Geometry: final body of the model. Coordinates: model frame, mm. A direction names the side the tool comes from. Round coordinates to 2 decimals unless told otherwise and drop trailing zeros. Loops run counter-clockwise (first coordinate to the right, second up) from the corner with the lowest first, then second, coordinate; pieces in that order, holes last. Notation, with made-up numbers: M 38,-26.75 L 64,-26.75 A31 ccw 64,-0.75 Z; hole C 34.25,-17 d1. An arc over 180 degrees is marked long. Write each question's results on one line, items separated by ' | '.
```python
from build123d import *

# Parameters (mm, degrees)
SZKIC1_W                         = 25.6
SZKIC1_H                         = 10
DODANIE_WYCI_GNI_CIE1_DEPTH      = 5
SZKIC2_R                         = 1.75
WYTNIJ_WYCI_GNI_CIE1_DEPTH       = 5
SZKIC3_W                         = 25.6
SZKIC3_H                         = 5
DODANIE_WYCI_GNI_CIE2_DEPTH      = 5
SZKIC4_W                         = 25.6
SZKIC4_H                         = 5
DODANIE_WYCI_GNI_CIE3_DEPTH      = 17
SZKIC5_R                         = 1.75
WYTNIJ_WYCI_GNI_CIE2_DEPTH       = 20
SZKIC6_W                         = 2
SZKIC6_H                         = 15
WYTNIJ_WYCI_GNI_CIE3_DEPTH       = 28.346663416
DODANIE_WYCI_GNI_CIE4_DEPTH      = 0.5
DODANIE_WYCI_GNI_CIE4_DEPTH_BACK = 7.5
SZKIC8_R                         = 1.75
WYTNIJ_WYCI_GNI_CIE4_DEPTH       = 48.531147682
SZKIC9_W                         = 37
SZKIC9_H                         = 6
DODANIE_WYCI_GNI_CIE5_DEPTH      = 20.5
SZKIC10_W                        = 37
SZKIC10_H                        = 6
SZKIC10_R                        = 1.75
DODANIE_WYCI_GNI_CIE6_DEPTH      = 5
SZKIC11_W                        = 16.1
SZKIC11_H                        = 5
DODANIE_WYCI_GNI_CIE7_DEPTH      = 15
SFAZOWANIE2_SIZE                 = 7.5
SFAZOWANIE2_SIZE2                = 2.009618943


with BuildPart() as part:
    # Szkic1 → Dodanie-wyciągnięcie1 (new body)
    with BuildSketch(Plane.XY):
        Rectangle(SZKIC1_W, SZKIC1_H)
    extrude(amount=DODANIE_WYCI_GNI_CIE1_DEPTH)

    # Szkic2 → Wytnij-wyciągnięcie1 (cut)
    with BuildSketch(Plane.XY.offset(5)):
        with Locations((-6, 0)):
            Circle(SZKIC2_R)
        with Locations((6, 0)):
            Circle(SZKIC2_R)
    extrude(amount=-WYTNIJ_WYCI_GNI_CIE1_DEPTH, mode=Mode.SUBTRACT)

    # Szkic3 → Dodanie-wyciągnięcie2 (add)
    with BuildSketch(Plane(origin=(0, 5, 0), x_dir=(1, 0, 0), z_dir=(0, 1, 0))):
        with Locations((0, -2.5)):
            Rectangle(SZKIC3_W, SZKIC3_H)
    extrude(amount=DODANIE_WYCI_GNI_CIE2_DEPTH)

    # Szkic4 → Dodanie-wyciągnięcie3 (add)
    with BuildSketch(Plane(origin=(0, 0, 0), x_dir=(-1, 0, 0), z_dir=(0, 0, -1))):
        with Locations((0, 7.5)):
            Rectangle(SZKIC4_W, SZKIC4_H)
    extrude(amount=DODANIE_WYCI_GNI_CIE3_DEPTH)

    # Szkic5 → Wytnij-wyciągnięcie2 (cut)
    with BuildSketch(Plane(origin=(0, 10, 0), x_dir=(1, 0, 0), z_dir=(0, 1, 0))):
        with Locations(Location((-0.8, 12, 0), (0, 0, 180))):
            Circle(SZKIC5_R)
    extrude(amount=-WYTNIJ_WYCI_GNI_CIE2_DEPTH, mode=Mode.SUBTRACT)

    # Szkic6 → Wytnij-wyciągnięcie3 (cut, through all)
    with BuildSketch(Plane.XY.offset(5)):
        with Locations((11.8, 2.5)):
            Rectangle(SZKIC6_W, SZKIC6_H)
    extrude(amount=-WYTNIJ_WYCI_GNI_CIE3_DEPTH, mode=Mode.SUBTRACT)

    # Szkic7 → Dodanie-wyciągnięcie4 (add, two sides: drawn at the far end of the back side and taken through both)
    with BuildSketch(Plane(origin=(10.8, 0, 0), x_dir=(0, 0, -1), z_dir=(1, 0, 0)).offset(-DODANIE_WYCI_GNI_CIE4_DEPTH_BACK)):
        Polygon((-5, 10), (17, 10), (17, 20), (-8, 40), (-16, 40), (-20, 25), (-20, 5), (-5, 5), align=None)
    extrude(amount=DODANIE_WYCI_GNI_CIE4_DEPTH + DODANIE_WYCI_GNI_CIE4_DEPTH_BACK)

    # Szkic8 → Wytnij-wyciągnięcie4 (cut, through all)
    with BuildSketch(Plane.ZY.offset(-3.3)):
        with Locations((12.5, 15)):
            Circle(SZKIC8_R)
        with Locations((12.5, 36.7)):
            Circle(SZKIC8_R)
        with Locations((-11.5, 15)):
            Circle(SZKIC8_R)
    extrude(amount=-WYTNIJ_WYCI_GNI_CIE4_DEPTH, mode=Mode.SUBTRACT)

    # Szkic9 → Dodanie-wyciągnięcie5 (add)
    with BuildSketch(Plane(origin=(10.8, 0, 0), x_dir=(0, 0, -1), z_dir=(1, 0, 0))):
        with Locations((-1.5, 8)):
            Rectangle(SZKIC9_W, SZKIC9_H)
    extrude(amount=DODANIE_WYCI_GNI_CIE5_DEPTH)

    # Szkic10 → Dodanie-wyciągnięcie6 (add)
    # profile 1 of 2: a face of its own
    with BuildSketch(Plane(origin=(31.3, 0, 0), x_dir=(0, 0, -1), z_dir=(1, 0, 0))):
        with Locations((-1.5, 8)):
            Rectangle(SZKIC10_W, SZKIC10_H)
    # profile 2 of 2: a face of its own
    with BuildSketch(Plane(origin=(31.3, 0, 0), x_dir=(0, 0, -1), z_dir=(1, 0, 0))):
        Polygon((-8, 40), (-16, 40), (-20, 25), (-20, 11), (17, 11), (17, 20), align=None)
        with Locations(Location((-12.5, 15, 0), (0, 0, 180))):
            Circle(SZKIC10_R, mode=Mode.SUBTRACT)
        with Locations(Location((-12.5, 36.7, 0), (0, 0, 180))):
            Circle(SZKIC10_R, mode=Mode.SUBTRACT)
        with Locations(Location((11.5, 15, 0), (0, 0, 180))):
            Circle(SZKIC10_R, mode=Mode.SUBTRACT)
    extrude(amount=DODANIE_WYCI_GNI_CIE6_DEPTH)

    # Szkic11 → Dodanie-wyciągnięcie7 (add)
    with BuildSketch(Plane.XY.offset(5)):
        with Locations((-4.75, 7.5)):
            Rectangle(SZKIC11_W, SZKIC11_H)
    extrude(amount=DODANIE_WYCI_GNI_CIE7_DEPTH)

    # Sfazowanie2
    sfazowanie2_edges = [part.edges().sort_by_distance(p)[0] for p in [
        (36.3, 5, 1.5),
    ]]
    sfazowanie2_side = [part.faces().sort_by_distance(p)[0] for p in [
        (12.712207968, 5, 1.507036511),
    ]]
    chamfer(sfazowanie2_edges, length=SFAZOWANIE2_SIZE, length2=SFAZOWANIE2_SIZE2, reference=sfazowanie2_side[0])


solid = part.part
```
1. Pin query (flat end, axial travel): P1, Ø8, axis at y = 29, z = 3, coming from the -X side; P2, Ø4, axis at x = -0.5, y = 18, coming from the +Z side; P3, Ø6, axis at x = -5, z = 7, coming from the +Y side; P4, Ø8, axis at x = 29, z = -11, coming from the -Y side. Return the tip coordinate at first contact, or that it passes through.
Answer key:
P1: stops at x = 3.3 | P2: passes through | P3: stops at y = 10 | P4: stops at y = 5
2. Access query for faces 1 (the face through (11.3, 22, 6)), 2 (the face through (36.3, 20, 6)). Directions: +Z, -Z, +X, -X, +Y, -Y. A direction counts if a zero-diameter tool reaches every point of the face in a straight line with its end or side. Return the directions, or none.
Answer key:
face 1: +Z, -Z, +Y | face 2: +Z, -Z, +X, +Y, -Y
3. Section A-A (x = 6). Output: boundary loops of the cut face in (y, z).
Answer key:
outline: M -5,0 L -1.75,0 L -1.75,5 L -5,5 Z; M 1.75,0 L 5,0 L 5,-17 L 20,-17 L 40,8 L 40,16 L 25,20 L 5,20 L 5,5 L 1.75,5 Z; hole C 15,-11.5 d3.5; hole C 15,12.5 d3.5; hole C 36.7,12.5 d3.5
4. Section C-C (z = -12). Output: boundary loops of the cut face in (x, y).
Answer key:
outline: M -12.8,5 L -2.55,5 L -2.55,10 L -12.8,10 Z; M 0.95,5 L 28.8,5 L 36.3,7.01 L 36.3,13.32 L 31.3,13.32 L 31.3,11 L 11.3,11 L 11.3,13.32 L 3.3,13.32 L 3.3,10 L 0.95,10 Z; M 3.3,16.68 L 11.3,16.68 L 11.3,24 L 3.3,24 Z; M 31.3,16.68 L 36.3,16.68 L 36.3,24 L 31.3,24 Z
5. Ray query, probe 1 along Z at (x, y) = (33.8, 15); probe 2 along Y at (x, z) = (5.5, 12.5); probe 3 along X at (y, z) = (34.5, 2). Return the intervals inside material, ascending.
Answer key:
probe 1: z = -17 to -13.25, -9.75 to 10.75, 14.25 to 20 | probe 2: y = 5 to 13.25, 16.75 to 34.95, 38.45 to 40 | probe 3: x = 3.3 to 11.3, 31.3 to 36.3
6. Section B-B (y = 15). Output: boundary loops of the cut face in (x, z), then the cut area to 3 significant figures.
Answer key:
outline: M 3.3,-17 L 11.3,-17 L 11.3,-13.25 L 3.3,-13.25 Z; M 3.3,-9.75 L 11.3,-9.75 L 11.3,10.75 L 3.3,10.75 Z; M 3.3,14.25 L 11.3,14.25 L 11.3,20 L 3.3,20 Z; M 31.3,-17 L 36.3,-17 L 36.3,-13.25 L 31.3,-13.25 Z; M 31.3,-9.75 L 36.3,-9.75 L 36.3,10.75 L 31.3,10.75 Z; M 31.3,14.25 L 36.3,14.25 L 36.3,20 L 31.3,20 Z | area: 390 mm²
7. Draft query along Y for faces 3 (the face through (7.24, 34.99, 12.12)), 4 (the face through (32.6, 6.02, 1.76)), 5 (the face through (3.3, 22, 6)). Return one class per face: pulls with the +Y half, pulls with the -Y half, needs draft (parallel to the pull), parting line crosses it, or undercut.
Answer key:
face 3: undercut | face 4: pulls with the -Y half | face 5: needs draft
8. Section D-D (x = -6). Output: boundary loops of the cut face in (y, z), then the cut area to 4 significant figures.
Answer key:
outline: M -5,0 L -1.75,0 L -1.75,5 L -5,5 Z; M 1.75,0 L 5,0 L 5,-17 L 10,-17 L 10,20 L 5,20 L 5,5 L 1.75,5 Z | area: 217.5 mm²
